Design review of the part built by this model. Coordinates are the model's own, in mm. A direction names the side the tool comes from. Round coordinates to 2 decimals unless told otherwise and drop trailing zeros. Order: outer loops, then holes, each group sorted by start corner. A loop starts at its lowest first (then second) coordinate and runs counter-clockwise, first axis right, second up. Notation, with made-up numbers: M 68,80.5 L 109,80.5 A21 cw 109,116.5 Z; hole C 4.5,-32 d5. An arc over 180 degrees is marked long. Write item = value, one per line. Start each with the question number.
```python
from build123d import *

# Parameters (mm, degrees)
EXTRUDE_1_DEPTH     = 1.25
EXTRUDE_2_DEPTH     = 2.5
SKETCH_3_R          = 0.6
CUT_EXTRUDE_1_DEPTH = 3.5
FILLET_1_R          = 0.5
SKETCH_5_W          = 5.025
SKETCH_5_H          = 1.95
CUT_EXTRUDE_2_DEPTH = 3.5
SKETCH_6_R          = 0.6
CUT_EXTRUDE_3_DEPTH = 3.5
CUT_EXTRUDE_4_DEPTH = 3.5
SKETCH_8_R          = 0.6
CUT_EXTRUDE_5_DEPTH = 3.5
FILLET_2_R          = 1
EXTRUDE_3_DEPTH     = 2.5
SKETCH_10_R         = 0.6
CUT_EXTRUDE_6_DEPTH = 3.5
FILLET_3_R          = 0.5
SKETCH_11_R         = 1.05
CUT_EXTRUDE_7_DEPTH = 3.5


with BuildPart() as part:
    # 草图2 → 凸台-拉伸1 (new body, symmetric)
    with BuildSketch(Plane(origin=(0, 0, 0), x_dir=(0, 0, -1), z_dir=(1, 0, 0))):
        Polygon((-5.025, 65), (-5.025, 8.5), (-8.025, 8.5), (-8.025, 3.5), (-5.025, 3.5), (-5.025, 2), (5.025, 2), (5.025, 3.5), (8.025, 3.5), (8.025, 8.5), (5.025, 8.5), (5.025, 65), align=None)
    extrude(amount=EXTRUDE_1_DEPTH, both=True)

    # 草图4 → 凸台-拉伸2 (add)
    with BuildSketch(Plane.ZY.offset(1.25)):
        Polygon((-5.025, 65), (-8.025, 10.95), (-5.025, 10.95), align=None)
    extrude(amount=-EXTRUDE_2_DEPTH)

    # 草图3 → 切除-拉伸1 (cut, through all)
    with BuildSketch(Plane(origin=(1.25, 0, 0), x_dir=(0, 0, -1), z_dir=(1, 0, 0))):
        with Locations((-5.025, 9.1)):
            Circle(SKETCH_3_R)
        with Locations((-5.625, 3.5)):
            Circle(SKETCH_3_R)
        with Locations((5.025, 9.1)):
            Circle(SKETCH_3_R)
        with Locations((5.625, 3.5)):
            Circle(SKETCH_3_R)
        with Locations((5.625, 10.95)):
            Circle(SKETCH_3_R)
    extrude(amount=-CUT_EXTRUDE_1_DEPTH, mode=Mode.SUBTRACT)

    # 圆角1
    fillet_1_edges = [part.edges().sort_by_distance(p)[0] for p in [
        (0, 8.5, -8.025),
        (0, 3.5, -8.025),
        (0, 2, -5.025),
        (0, 2, 5.025),
        (0, 3.5, 8.025),
        (0, 8.5, 8.025),
        (0, 10.95, -8.025),
    ]]
    fillet(fillet_1_edges, radius=FILLET_1_R)

    # 草图5 → 切除-拉伸2 (cut, through all)
    with BuildSketch(Plane(origin=(1.25, 0, 0), x_dir=(0, 0, -1), z_dir=(1, 0, 0))):
        with Locations((-2.5125, 38.475)):
            Rectangle(SKETCH_5_W, SKETCH_5_H)
        with Locations((-2.5125, 60.525)):
            Rectangle(SKETCH_5_W, SKETCH_5_H)
    extrude(amount=-CUT_EXTRUDE_2_DEPTH, mode=Mode.SUBTRACT)

    # 草图6 → 切除-拉伸3 (cut, through all)
    with BuildSketch(Plane(origin=(1.25, 0, 0), x_dir=(0, 0, -1), z_dir=(1, 0, 0))):
        with Locations((-0.6, 61.5)):
            Circle(SKETCH_6_R)
        with Locations((-0.6, 59.55)):
            Circle(SKETCH_6_R)
        with Locations((-0.6, 39.45)):
            Circle(SKETCH_6_R)
        with Locations((-0.6, 37.5)):
            Circle(SKETCH_6_R)
    extrude(amount=-CUT_EXTRUDE_3_DEPTH, mode=Mode.SUBTRACT)

    # 草图7 → 切除-拉伸4 (cut, through all)
    with BuildSketch(Plane.ZY.offset(1.25)):
        Polygon((-5.025, 65), (-5.025, 30), (-6.967645698, 30), align=None)
    extrude(amount=-CUT_EXTRUDE_4_DEPTH, mode=Mode.SUBTRACT)

    # 草图8 → 切除-拉伸5 (cut, through all)
    with BuildSketch(Plane.ZY.offset(1.25)):
        with Locations((-5.025, 30.6)):
            Circle(SKETCH_8_R)
    extrude(amount=-CUT_EXTRUDE_5_DEPTH, mode=Mode.SUBTRACT)

    # 圆角2
    fillet_2_edges = [part.edges().sort_by_distance(p)[0] for p in [
        (0, 65, -5.025),
        (0, 30, -6.967645698),
        (0, 65, 5.025),
    ]]
    fillet(fillet_2_edges, radius=FILLET_2_R)

    # 草图9 → 凸台-拉伸3 (add)
    with BuildSketch(Plane.ZY.offset(1.25)):
        Polygon((5.025, 59.55), (10, 59.55), (10, 61.35), (15, 60.010254038), (15, 57.010254038), (5.025, 54.55), align=None)
        Polygon((15, 41.989745962), (5.025, 44.45), (5.025, 39.45), (10, 39.45), (10, 37.65), (15, 38.989745962), align=None)
    extrude(amount=-EXTRUDE_3_DEPTH)

    # 草图10 → 切除-拉伸6 (cut, through all)
    with BuildSketch(Plane.ZY.offset(1.25)):
        with Locations((5.025, 53.95)):
            Circle(SKETCH_10_R)
        with Locations((5.025, 45.05)):
            Circle(SKETCH_10_R)
        with Locations((9.4, 59.55)):
            Circle(SKETCH_10_R)
        with Locations((9.4, 39.45)):
            Circle(SKETCH_10_R)
    extrude(amount=-CUT_EXTRUDE_6_DEPTH, mode=Mode.SUBTRACT)

    # 圆角3
    fillet_3_edges = [part.edges().sort_by_distance(p)[0] for p in [
        (0, 61.35, 10),
        (0, 60.010254038, 15),
        (0, 57.010254038, 15),
        (0, 41.989745962, 15),
        (0, 38.989745962, 15),
        (0, 37.65, 10),
    ]]
    fillet(fillet_3_edges, radius=FILLET_3_R)

    # 草图11 → 切除-拉伸7 (cut, through all)
    with BuildSketch(Plane(origin=(1.25, 0, 0), x_dir=(0, 0, -1), z_dir=(1, 0, 0))):
        with Locations((-0.475, 27.5)):
            Circle(SKETCH_11_R)
    extrude(amount=-CUT_EXTRUDE_7_DEPTH, mode=Mode.SUBTRACT)


solid = part.part
```
(1) Insertion check: pin 1 (0.8 mm diameter, centred on x = -0.5, y = 7, fed in from +Z) (3 decimals); pin 2 (1 mm diameter, centred on x = 0, z = 7, fed in from -Y); pin 3 (1.3 mm diameter, centred on x = -0.5, y = 39, fed in from -Z) (3 decimals); pin 4 (1.9 mm diameter, centred on y = 27.5, z = 0.475, fed in from +X). Each pin has a flat end and moves straight along its axis. Give the tip position at first contact, or say it passes through.
(2) For line 1 along Y through (x, z) = (-0.35, 5.5); line 2 along Y through (x, z) = (0.6, 7); line 3 along Y through (x, z) = (0.75, 10.5), list the stretches that pass through material, from the lowest coordinate up. Write a range as [from, to].
(3) Draft analysis for pull direction Y (two halves, no side actions). For faces 1 (the face through (0, 39.45, 5)), 2 (the face through (0, 60, 10)), 3 (the face through (-0.018, 60.653, 12.601)), state which applies: pulls with the +Y half, pulls with the -Y half, needs draft (parallel to the pull), parting line crosses it, or undercut.
(4) For faces 4 (the face through (0, 48, -5.025)), 5 (the face through (0, 63, 5.025)), 6 (the face through (0, 8.5, -6)), list the 3-axis set-ups (+Z, -Z, +X, -X, +Y, -Y) from which the entire face can be reached by the end or side of a thin tool; tool diameter is ignored.
(5) Consider section B-B, the plane y = 27.5. Write out the cut boundary in (x, z) (3 decimals).
(6) Consider section A-A, the plane z = 13.25. Write out the cut boundary in (x, y), then the cut area to 3 significant figures.
(7) Consider section C-C, the plane y = 36. Write out the cut boundary in (x, z) (3 decimals), then the cut area to 3 significant figures.
(8) Consider section D-D, the plane y = 53.95. Write out the cut boundary in (x, z) (3 decimals).
Completed:
q1.pin_1 = 8.025
q1.pin_2 = 3.5
q1.pin_3 = -5.025
q1.pin_4 = through
q2.line_1 = [4.09, 8.5], [39.45, 44.33], [54.67, 59.55]
q2.line_2 = [3.5, 8.5], [39.45, 43.96], [55.04, 59.55]
q2.line_3 = [37.8, 43.1], [55.9, 61.2]
q3.face_1 = undercut
q3.face_2 = needs draft
q3.face_3 = pulls with the +Y half
q4.face_4 = -Z, +X, -X, +Y
q4.face_5 = +Z, +X, -X, +Y
q4.face_6 = -Z, +X, -X
q5.outline = M -1.25,-7.106 L 1.25,-7.106 L 1.25,-0.575 L -1.25,-0.575 Z; M -1.25,1.525 L 1.25,1.525 L 1.25,5.025 L -1.25,5.025 Z
q6.outline = M -1.25,38.52 L 1.25,38.52 L 1.25,42.42 L -1.25,42.42 Z; M -1.25,56.58 L 1.25,56.58 L 1.25,60.48 L -1.25,60.48 Z
q6.area = 19.5 mm2
q7.outline = M -1.25,-5.025 L 1.25,-5.025 L 1.25,5.025 L -1.25,5.025 Z
q7.area = 25.1 mm2
q8.outline = M -1.25,-5.025 L 1.25,-5.025 L 1.25,4.425 L -1.25,4.425 Z
